Geometry check sheet. Reference: drawing and pictorial views, mm from the part's lowest x, y, z. Give positions to 0.01 mm unless a question says otherwise; leave off trailing zeros. Write each loop counter-clockwise with the first axis right and the second up, starting at its lowest first coordinate (ties: lowest second). Pieces come first, ordered by that corner, then holes. Notation, with made-up numbers: (4, 43) - (9, 43) arc R15 ccw to (9, 64) - close; hole circle Ø7 at (14.25, 41.5). An arc over 180 degrees is marked (long way). Put each result on its own line as item: value.
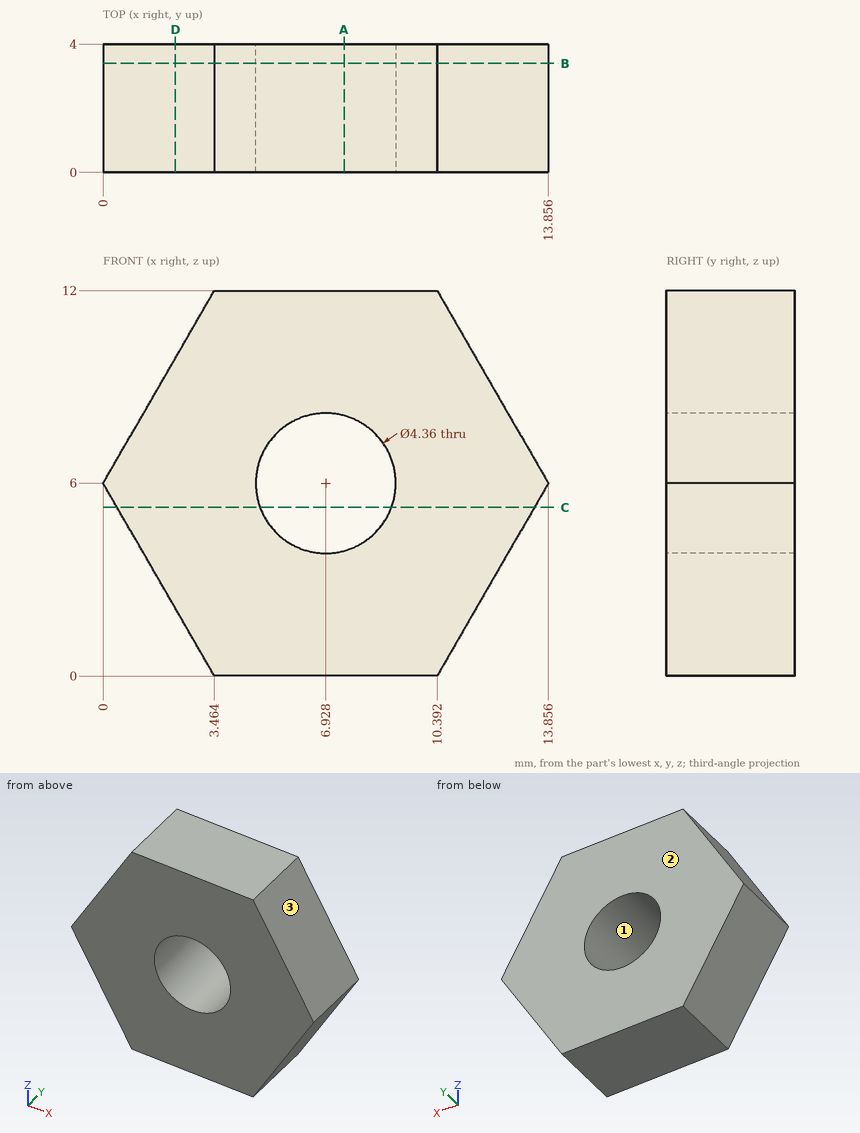
Q1. Section check A-A, the plane x = 7.5. Record the cut outline in (y, z).
Answers follow:
outline: (0, 0) - (4, 0) - (4, 3.9) - (0, 3.9) - close; (0, 8.1) - (4, 8.1) - (4, 12) - (0, 12) - close
Q2. Section check B-B, the plane y = 3.4. Record the cut outline in (x, z), plus the area to 3 significant figures.
Answers follow:
outline: (0, 6) - (3.46, 0) - (10.39, 0) - (13.86, 6) - (10.39, 12) - (3.46, 12) - close; hole circle Ø4.36 at (6.93, 6)
area: 110 mm2
Q3. Section check C-C, the plane z = 5.25. Record the cut outline in (x, y) (1 decimal).
Answers follow:
outline: (0.4, 0) - (4.9, 0) - (4.9, 4) - (0.4, 4) - close; (9, 0) - (13.4, 0) - (13.4, 4) - (9, 4) - close
Q4. Go/stop test with a flat-tipped pin: pin 1 Ø1 at (y, z) = (3, 4.5) entering from +X. Record where the tip stops, or that it passes through.
Answers follow:
pin 1: stops at x = 13.28
Q5. Section check D-D, the plane x = 2.25. Record the cut outline in (y, z).
Answers follow:
outline: (0, 2.1) - (4, 2.1) - (4, 9.9) - (0, 9.9) - close
Q6. Release check for a two-part mould opening along Z. For the marked faces 1, 2 and 3 record: released by +Z, released by -Z, zero draft, split by the parting line, or undercut.
Answers follow:
face 1: undercut
face 2: zero draft
face 3: released by +Z
Q7. Scan lines: line 1 along Z through (x, y) = (7, 2.8); line 2 along Z through (x, y) = (5.75, 2.4) (1 decimal); line 3 along X through (y, z) = (0.4, 7.25) (1 decimal). Record each from-to range of solid material in increasing order.
Answers follow:
line 1: z = 0 to 3.82, 8.18 to 12
line 2: z = 0 to 4.2, 7.8 to 12
line 3: x = 0.7 to 5.1, 8.7 to 13.1
